Part model, mm, in its own coordinate system. A direction names the side the tool comes from. Coordinates: 2 decimals unless noted, no trailing zeros. Loops run counter-clockwise (first coordinate to the right, second up) from the corner with the lowest first, then second, coordinate; pieces in that order, holes last. Notation, with made-up numbers: (-12.75, 9) -> (36.25, 9) arc R28 ccw to (36.25, 36) -> close; hole circle Ø8 at (-10, 53). An arc over 180 degrees is marked (long way). Use one line per item in the form item = value. Start each with the question number.
(1) Band-saw the part on A-A on y = -185. Give the cut face in (x, z), then the cut area to 3 significant figures.
(2) Mould opens along X. For faces 1 (the flat face through (240, -96, 2)), 2 (the flat face through (0, -96, 2)), 3 (the cylindrical face through (12.21, -7.97, 2.46)) say: +X half, -X half, draft (parallel to the pull), parting line (faces both ways), or undercut.
(3) Band-saw the part on B-B on z = 1.6. Give the cut face in (x, y), then the cut area to 3 significant figures.
(4) 3-axis set-ups, long thin cutter, end or side, ignore diameter. For faces 4 (the flat face through (155, -76, 3)), 5 (the flat face through (118, -94, 5)): which of +Z, -Z, +X, -X, +Y, -Y reach the whole face in a straight line?
(5) Drill centre lines: L1, parallel to Y at x = 10, z = 1.1; L2, parallel to X at y = -135.5, z = 3.1. Where is each one in solid material? Low to high. Write a range as [from, to].
(6) Band-saw the part on C-C on x = 10. Give the cut face in (y, z), then the cut area to 3 significant figures.
(7) Band-saw the part on D-D on y = -129. Give the cut face in (x, z), then the cut area to 3 significant figures.
(8) Pin check, flat tip, straight feed: P1, Ø2.5, axis at x = 159, z = 1.5, coming from the +Y side. Stop position of the tip, or through.
```python
from build123d import *

# Parameters (mm, degrees)
ESQUISSE1_W             = 240
ESQUISSE1_H             = 190
BOSS_EXTRU_1_DEPTH      = 5
ESQUISSE2_W             = 10
ESQUISSE2_H             = 150
ENL_V_MAT_EXTRU_1_DEPTH = 5
ESQUISSE3_R             = 3
ENL_V_MAT_EXTRU_2_DEPTH = 10


with BuildPart() as part:
    # Esquisse1 → Boss.-Extru.1 (new body)
    with BuildSketch(Plane.XY):
        with Locations((120, -95)):
            Rectangle(ESQUISSE1_W, ESQUISSE1_H)
    extrude(amount=BOSS_EXTRU_1_DEPTH)

    # Esquisse2 → Enlèv. mat.-Extru.1 (cut)
    with BuildSketch(Plane.XY.offset(5)):
        with Locations((160, -75)):
            Rectangle(ESQUISSE2_W, ESQUISSE2_H)
    extrude(amount=-ENL_V_MAT_EXTRU_1_DEPTH, mode=Mode.SUBTRACT)

    # Esquisse3 → Enlèv. mat.-Extru.2 (cut)
    with BuildSketch(Plane(origin=(0, 0, 0), x_dir=(-1, 0, 0), z_dir=(0, 0, -1))):
        with Locations((-10, -185)):
            Circle(ESQUISSE3_R)
        with Locations((-10, -10)):
            Circle(ESQUISSE3_R)
        with Locations(Location((-230, -185, 0), (0, 0, 180))):
            Circle(ESQUISSE3_R)
        with Locations(Location((-230, -10, 0), (0, 0, 180))):
            Circle(ESQUISSE3_R)
    extrude(amount=-ENL_V_MAT_EXTRU_2_DEPTH, mode=Mode.SUBTRACT)


solid = part.part
```
A:
q1.outline = (0, 0) -> (7, 0) -> (7, 5) -> (0, 5) -> close; (13, 0) -> (227, 0) -> (227, 5) -> (13, 5) -> close; (233, 0) -> (240, 0) -> (240, 5) -> (233, 5) -> close
q1.area = 1,140 mm²
q2.face_1 = +X half
q2.face_2 = -X half
q2.face_3 = undercut
q3.outline = (0, -190) -> (240, -190) -> (240, 0) -> (165, 0) -> (165, -150) -> (155, -150) -> (155, 0) -> (0, 0) -> close; hole circle Ø6 at (10, -185); hole circle Ø6 at (10, -10); hole circle Ø6 at (230, -185); hole circle Ø6 at (230, -10)
q3.area = 44,000 mm²
q4.face_4 = +Z, -Z, +Y
q4.face_5 = +Z, +X, -X, +Y, -Y
q5.L1 = [-190, -188], [-182, -13], [-7, 0]
q5.L2 = [0, 155], [165, 240]
q6.outline = (-190, 0) -> (-188, 0) -> (-188, 5) -> (-190, 5) -> close; (-182, 0) -> (-13, 0) -> (-13, 5) -> (-182, 5) -> close; (-7, 0) -> (0, 0) -> (0, 5) -> (-7, 5) -> close
q6.area = 890 mm²
q7.outline = (0, 0) -> (155, 0) -> (155, 5) -> (0, 5) -> close; (165, 0) -> (240, 0) -> (240, 5) -> (165, 5) -> close
q7.area = 1,150 mm²
q8.P1 = -150
